Can you work these out from the model? Positions are in its coordinate system, mm. Face numbers are marked on the shaded views. A direction names the side the tool comes from. Coordinates: 2 decimals unless noted, no trailing zeros. Order: outer loops, then holes, each group sorted by start corner. A loop starts at its lowest first (then second) coordinate and runs counter-clockwise, first axis right, second up.
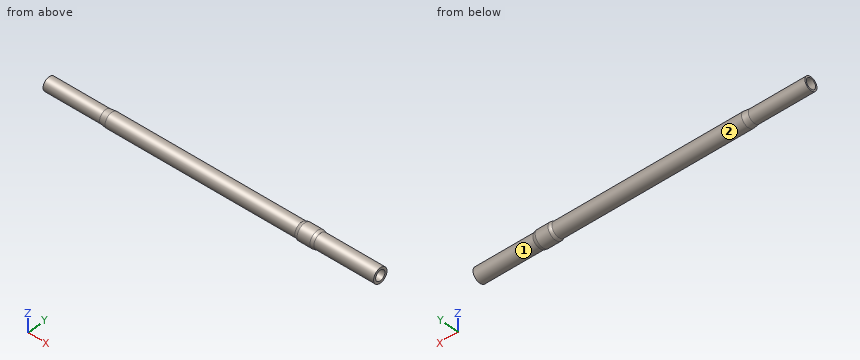
```python
from build123d import *

# Parameters (mm, degrees)
F0_W = 5.08
F0_H = 0.5969
F3_D = 0.9144


# Not quite as in the source:
# - a fillet or chamfer that OpenCascade refuses, or shapes differently, is made with other operations: its cross-section is extruded or revolved along the edge and cut away or added


with BuildPart() as f1:
    # F0 (on Front) → F1 (revolve)
    with BuildSketch(Plane.XZ):
        with Locations((2.54, 0.29845)):
            Rectangle(F0_W, F0_H)
        Polygon((5.6251967326, 0.6604), (5.6251967326, 0), (29.718, 0), (29.718, 0.6604), (24.3530571461, 0.6604), (24.3530571461, 0.7366), (22.6445570588, 0.7366), (22.6431967326, 0.6604), align=None)
        Polygon((5.08, 0.5969), (5.08, 0), (5.6251967326, 0), (5.6251967326, 0.6604), align=None)
    revolve(axis=Axis((14.859, 0, 0), (1, 0, 0)))

    # F3 (through all)
    with Locations(Plane(origin=(0, 0, 0), x_dir=(0, 1, 0), z_dir=(-1, 0, 0))):
        with Locations((0, 0)):
            Hole(F3_D / 2)

    # F4: fillet of radius 0.5588 on 1 edges, made by hand

    # F4_s1 → F4_t2 (revolve, cut)
    with BuildSketch(Plane.XZ):
        with BuildLine():
            ThreePointArc((24.3530571461, 0.6604), (24.21726941, 0.7172137188), (24.0713575188, 0.7366))
            Line((24.0713575188, 0.7366), (24.3530571461, 0.7366))
            Line((24.3530571461, 0.7366), (24.3530571461, 0.6604))
        make_face()
    revolve(axis=Axis((24.3530571461, 0, 0), (1, 0, 0)), mode=Mode.SUBTRACT)

    # F5: fillet of radius 0.5588 on 1 edges, made by hand

    # F5_s1 → F5_t2 (revolve, cut)
    with BuildSketch(Plane.XZ):
        with BuildLine():
            ThreePointArc((22.6431967326, 0.6604), (22.7789844686, 0.7172137188), (22.9248963599, 0.7366))
            Line((22.9248963599, 0.7366), (22.6445570588, 0.7366))
            Line((22.6445570588, 0.7366), (22.6431967326, 0.6604))
        make_face()
    revolve(axis=Axis((22.6445570588, 0, 0), (1, 0, 0)), mode=Mode.SUBTRACT)


solid = f1.part
```
1. On a 3-axis mill with a long thin cutter (end or side, diameter ignored), from which of +Z, -Z, +X, -X, +Y, -Y can I reach the whole of each face in a straight line? I mean the marked faces 1 and 2. Say none if no direction works.
Completed:
face 1: +X
face 2: -X
2. Imagine slicing it at A-A on x = 3.25. Please give me the cut outline in (y, z), then the cut area to 3 significant figures.
Completed:
outline: circle Ø1.19 at (0, 0); hole circle Ø0.91 at (0, 0)
area: 0.463 mm2
3. Imagine slicing it at B-B on x = 16.75. Please give me the cut outline in (y, z).
Completed:
outline: circle Ø1.32 at (0, 0); hole circle Ø0.91 at (0, 0)
4. Please list where these lines run through material, in increasing order: probe 1 along Z at (x, y) = (22, 0); probe 2 along Y at (x, z) = (5.5, -0.3) (3 decimals); probe 3 along Y at (x, z) = (12.5, 0.15).
Completed:
probe 1: z = -0.66 to -0.46, 0.46 to 0.66
probe 2: y = -0.572 to -0.345, 0.345 to 0.572
probe 3: y = -0.64 to -0.43, 0.43 to 0.64
